Build history of the part. All positions in model axes, mm. Round coordinates to 2 decimals unless told otherwise and drop trailing zeros. Loops run counter-clockwise (first coordinate to the right, second up) from the corner with the lowest first, then second, coordinate; pieces in that order, holes last. Notation, with made-up numbers: (79.5, 1.25) - (130.5, 1.25) arc R24 ccw to (130.5, 21.25) - close; hole circle Ø11 at (66.5, 34.5). An arc over 180 degrees is marked (long way). Use a Markdown table: item, result.
from build123d import *

# Parameters (mm, degrees)
F0_W     = 75
F0_H     = 35
F1_DEPTH = 10.57
F2_D     = 11
F3_R     = 1


with BuildPart() as f1:
    # F0 (on Top) → F1 (new body)
    with BuildSketch(Plane.XY):
        Rectangle(F0_W, F0_H)
    extrude(amount=F1_DEPTH)

    # F2 (through all)
    with Locations(Plane(origin=(0, 0, 0), x_dir=(1, 0, 0), z_dir=(0, 0, -1))):
        with Locations((-18.75, 0), (18.75, 0)):
            Hole(F2_D / 2)

    # F3
    f3_edges = [f1.edges().sort_by_distance(p)[0] for p in [
        (0, -17.5, 0),
        (-37.5, -17.5, 5.285),
        (37.5, -17.5, 5.285),
        (37.5, 0, 0),
        (-37.5, 0, 0),
        (0, 17.5, 0),
        (-37.5, 17.5, 5.285),
        (37.5, 17.5, 5.285),
    ]]
    fillet(f3_edges, radius=F3_R)


solid = f1.part
Q1. Cut at A-A, the plane x = -18.75. List the corners of the cut face in (y, z), plus the area to 3 significant figures.
Results found:
| item | result |
|---|---|
| outline | (-17.5, 1) arc R1 ccw to (-16.5, 0) - (-5.5, 0) - (-5.5, 10.57) - (-17.5, 10.57) - close; (5.5, 0) - (16.5, 0) arc R1 ccw to (17.5, 1) - (17.5, 10.57) - (5.5, 10.57) - close |
| area | 253 mm2 |
Q2. Cut at C-C, the plane z = 5.25. List the corners of the cut face in (x, y), plus the area to 3 significant figures.
Results found:
| item | result |
|---|---|
| outline | (-37.5, -16.5) arc R1 ccw to (-36.5, -17.5) - (36.5, -17.5) arc R1 ccw to (37.5, -16.5) - (37.5, 16.5) arc R1 ccw to (36.5, 17.5) - (-36.5, 17.5) arc R1 ccw to (-37.5, 16.5) - close; hole circle Ø11 at (-18.75, 0); hole circle Ø11 at (18.75, 0) |
| area | 2,430 mm2 |
Q3. Cut at D-D, the plane y = -3.5. List the corners of the cut face in (x, z).
Results found:
| item | result |
|---|---|
| outline | (-37.5, 1) arc R1 ccw to (-36.5, 0) - (-22.99, 0) - (-22.99, 10.57) - (-37.5, 10.57) - close; (-14.51, 0) - (14.51, 0) - (14.51, 10.57) - (-14.51, 10.57) - close; (22.99, 0) - (36.5, 0) arc R1 ccw to (37.5, 1) - (37.5, 10.57) - (22.99, 10.57) - close |
Q4. Pull direction Y, two halves, no side cores. Call faces 1 (the face through (-23.83, 2.11, 5.36)), 2 (the face through (-1, 17.5, 6)), 3 (the face through (13.67, 2.11, 5.36)), 4 (the face through (-1, 0, 10.57)): pulls with the +Y half, pulls with the -Y half, needs draft (parallel to the pull), parting line crosses it, or undercut.
Results found:
| item | result |
|---|---|
| face 1 | undercut |
| face 2 | pulls with the +Y half |
| face 3 | undercut |
| face 4 | needs draft |
Q5. Cut at B-B, the plane y = 0. List the corners of the cut face in (x, z).
Results found:
| item | result |
|---|---|
| outline | (-37.5, 1) arc R1 ccw to (-36.5, 0) - (-24.25, 0) - (-24.25, 10.57) - (-37.5, 10.57) - close; (-13.25, 0) - (13.25, 0) - (13.25, 10.57) - (-13.25, 10.57) - close; (24.25, 0) - (36.5, 0) arc R1 ccw to (37.5, 1) - (37.5, 10.57) - (24.25, 10.57) - close |
Q6. Probe line 1 (X direction, y = -0.5, z = 7.5); line 2 (Y direction, x = 18.75, z = 8.25); line 3 (Y direction, x = -21.5, z = 1). List the from-to ranges inside material, lowest first.
Results found:
| item | result |
|---|---|
| line 1 | x = -37.5 to -24.23, -13.27 to 13.27, 24.23 to 37.5 |
| line 2 | y = -17.5 to -5.5, 5.5 to 17.5 |
| line 3 | y = -17.5 to -4.76, 4.76 to 17.5 |
